The model under review builds one solid part; all positions refer to its coordinate system, in mm. A direction names the side the tool comes from. Coordinates: 2 decimals unless noted, no trailing zeros. Loops run counter-clockwise (first coordinate to the right, second up) from the corner with the lowest first, then second, coordinate; pieces in that order, holes last. Notation, with made-up numbers: M 3,71 L 40,71 A29 cw 40,93 Z; hole C 67,-18.5 d7. An arc over 180 degrees is marked long. Return JSON: item names as keys, results as strings.
```python
from build123d import *

# Parameters (mm, degrees)
SKETCH1_R                        = 76.2
BOSS_EXTRUDE1_DEPTH              = 114.3
CBORE_FOR_M10_SBHCS1_D           = 12
CBORE_FOR_M10_SBHCS1_CBORE_D     = 18.5
CBORE_FOR_M10_SBHCS1_CBORE_DEPTH = 5.5
CIRPATTERN1_COUNT                = 6


with BuildPart() as part:
    # Sketch1 → Boss-Extrude1 (new body)
    with BuildSketch(Plane(origin=(0, 0, 0), x_dir=(1, 0, 0), z_dir=(0, 1, 0))):
        Circle(SKETCH1_R)
    extrude(amount=BOSS_EXTRUDE1_DEPTH)

    # CBORE for M10 SBHCS1 (through all)
    with Locations(Plane(origin=(0, 114.3, 0), x_dir=(1, 0, 0), z_dir=(0, 1, 0))):
        with Locations((0, 50), (43.301270189, 25), (43.301270189, -25), (0, -50), (-43.301270189, -25), (-43.301270189, 25)):
            CounterBoreHole(CBORE_FOR_M10_SBHCS1_D / 2, CBORE_FOR_M10_SBHCS1_CBORE_D / 2, CBORE_FOR_M10_SBHCS1_CBORE_DEPTH)

    # Sketch47 → Tap Drill for M10 Helicoil1 (revolve, cut)
    with BuildSketch(Plane(origin=(55.7, 114.3, 0), x_dir=(0, 0, 1), z_dir=(1, 0, 0))):
        Polygon((0, 0), (0, 28.15451825), (5.25, 25), (5.25, 0), align=None)
    tap_drill_for_m10_helicoil1 = revolve(axis=Axis((55.7, 120.65, 0), (0, -1, 0)), mode=Mode.SUBTRACT)

    # CirPattern1: Tap Drill for M10 Helicoil1 ×6 about axis
    cirpattern1_axis = Axis((0, 0, 0), (0, 1, 0))
    for i in range(1, CIRPATTERN1_COUNT):
        add(tap_drill_for_m10_helicoil1.rotate(cirpattern1_axis, i * 360 / CIRPATTERN1_COUNT), mode=Mode.SUBTRACT)


solid = part.part
```
1. To check wall thickness, follow line 1 (Z direction, x = 0, y = 113); line 2 (Z direction, x = 4.5, y = 16.5); line 3 (X direction, y = 95, z = 1). State the ranges of each line that lie inside material, in increasing order.
Check values:
{"line 1": "-76.2 to -59.25, -40.75 to 40.75, 59.25 to 76.2", "line 2": "-76.07 to -53.97, -46.03 to 46.03, 53.97 to 76.07", "line 3": "-76.19 to -60.85, -50.55 to 50.55, 60.85 to 76.19"}
2. Add section A-A on x = 0. Give the boundary of the cut face in (y, z).
Check values:
{"outline": "M 0,-76.2 L 114.3,-76.2 L 114.3,-59.25 L 108.8,-59.25 L 108.8,-56 L 0,-56 Z; M 0,-44 L 108.8,-44 L 108.8,-40.75 L 114.3,-40.75 L 114.3,40.75 L 108.8,40.75 L 108.8,44 L 0,44 Z; M 0,56 L 108.8,56 L 108.8,59.25 L 114.3,59.25 L 114.3,76.2 L 0,76.2 Z"}
3. Add section D-D on x = 19.5. Give the boundary of the cut face in (y, z), plus the area to 3 significant figures.
Check values:
{"outline": "M 0,-73.66 L 114.3,-73.66 L 114.3,73.66 L 0,73.66 Z", "area": "16,800 mm²"}
4. Machinability: for faces 4 (the face through (37.76, 53.64, -22.7)), 5 (the face through (2, 108.8, 56)), which of the approach directions +Z, -Z, +X, -X, +Y, -Y give a long, thin tool a straight path to every point of the face, cutting with its end or side? Answer none if there is none.
Check values:
{"face 4": "+Y, -Y", "face 5": "+Y"}
5. Insertion check: pin 1 Ø9 at (x, z) = (-40, 26.5) entering from +Y; pin 2 Ø8 at (y, z) = (81.5, -12.5) entering from +X; pin 3 Ø5 at (x, y) = (7.5, 69.5) entering from -Z. Each pin has a flat end and moves straight along its axis. Give the tip position at first contact, or say it passes through.
Check values:
{"pin 1": "y = 108.8", "pin 2": "x = 75.72", "pin 3": "z = -76.04"}
6. The part is to be moulded in two halves that separate along Z. For faces 1 (the face through (22.725, 101.975, -47.1)), 2 (the face through (-1, 0, -1)), 3 (the face through (-60.47, 56.35, 46.367)), say which applies: released by +Z, released by -Z, zero draft, split by the parting line, or undercut.
Check values:
{"face 1": "undercut", "face 2": "zero draft", "face 3": "split by the parting line"}
7. Add section B-B on z = 22. Give the boundary of the cut face in (x, y), plus the area to 3 significant figures.
Check values:
{"outline": "M -72.96,0 L -48.5,0 L -48.5,108.8 L -52.05,108.8 L -52.05,114.3 L -72.96,114.3 Z; M -38.11,0 L 38.11,0 L 38.11,108.8 L 34.55,108.8 L 34.55,114.3 L -34.55,114.3 L -34.55,108.8 L -38.11,108.8 Z; M 48.5,0 L 72.96,0 L 72.96,114.3 L 52.05,114.3 L 52.05,108.8 L 48.5,108.8 Z", "area": "14,200 mm²"}
8. Add section C-C on y = 14. Give the boundary of the cut face in (x, z).
Check values:
{"outline": "C 0,0 d152.4; hole C -43.3,-25 d12; hole C -43.3,25 d12; hole C 0,-50 d12; hole C 0,50 d12; hole C 43.3,-25 d12; hole C 43.3,25 d12"}
